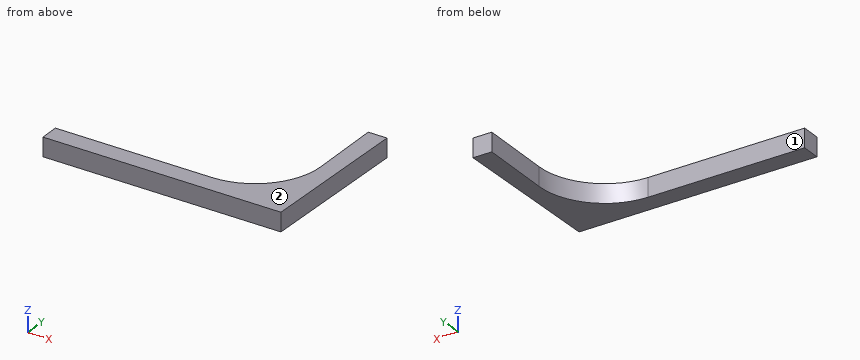
Autodesk Inventor part; units mm, degrees
ref_plane "YZ Plane" through (0, 0, 0) normal (1, 0, 0) x (0, 1, 0)
ref_plane "XZ Plane" through (0, 0, 0) normal (0, 1, 0) x (-1, 0, 0)
ref_plane "XY Plane" through (0, 0, 0) normal (0, 0, 1) x (1, 0, 0)
sketch "Sketch1" plane through (0, 0, 0) normal (0, 0, 1) x (1, 0, 0)
  circle A0 centre (0, 0) radius 21
  line L0 (0, -21) -> (-50, -21)
  line L1 (-50, -21) -> (-50, -27)
  line L2 (-50, -27) -> (49, -27)
  line L3 (21, 0) -> (21, 23)
  line L4 (21, 23) -> (27, 23)
  line L5 (27, 23) -> (26, -27)
  dimension "d0" = 42
  dimension "d1" = 50
  dimension "d2" = 6
  dimension "d4" = 6
  dimension "d5" = 50
extrude "Extrusion1" add sketch "Sketch1" along normal blind 6 contours L3 L4 L5 L2 L1 L0 A0
properties part number "hOLD_2"
Input: part model. Units: mm. Frame: model coordinates. Face numbers are marked on the shaded views. A direction names the side the tool comes from. Round coordinates to 2 decimals unless told otherwise and drop trailing zeros. Write each loop counter-clockwise with the first axis right and the second up, starting at its lowest first coordinate (ties: lowest second). Pieces come first, ordered by that corner, then holes. Notation, with made-up numbers: (13, -16) - (55, -16) arc R24 cw to (55, 15) - close; hole circle Ø2 at (-14.75, 69). An arc over 180 degrees is marked (long way). Write item = value, one per line.
(1) Section query B-B on y = 3.5. Output: boundary loops of the cut face in (x, z).
Geometry check:
outline = (21, 0) - (26.61, 0) - (26.61, 6) - (21, 6) - close
(2) Section query C-C on x = -9. Output: boundary loops of the cut face in (y, z), then the cut area to 3 significant figures.
Geometry check:
outline = (-27, 0) - (-21, 0) - (-21, 6) - (-27, 6) - close
area = 36.0 mm^2
(3) Access query for the marked faces 1 and 2. Directions: +Z, -Z, +X, -X, +Y, -Y. A direction counts if a zero-diameter tool reaches every point of the face in a straight line with its end or side. Return the directions, or none.
Geometry check:
face_1 = +Z, -Z, -X, +Y
face_2 = +Z, +X, -X, +Y, -Y
(4) Material intervals for probe 1 along Y at (x, z) = (-3, 3); probe 2 along X at (y, z) = (-18, 0.4); probe 3 along X at (y, z) = (8, 5.35), sorted ascending.
Geometry check:
probe_1 = -27 to -21
probe_2 = 10.82 to 26.18
probe_3 = 21 to 26.7
(5) Contact query for flat-ended pins moving along their axis: pin 1 Ø3 at (x, z) = (-21, 1.5) entering from +Y; pin 2 Ø2 at (x, y) = (-39.5, -19) entering from -Z; pin 3 Ø1.5 at (y, z) = (14.5, 3) entering from -X. Output: stop coordinate, or through.
Geometry check:
pin_1 = -21
pin_2 = through
pin_3 = 21
(6) Section query A-A on z = 2.95. Output: boundary loops of the cut face in (x, y), then the cut area to 3 significant figures.
Geometry check:
outline = (-50, -27) - (26, -27) - (27, 23) - (21, 23) - (21, 0) arc R21 cw to (0, -21) - (-50, -21) - close
area = 796 mm^2
